```python
from build123d import *

# Parameters (mm, degrees)
SKETCH2_R            = 2
BOSS_EXTRUDE1_DEPTH  = 28
SKETCH3_R            = 3
BOSS_EXTRUDE2_DEPTH  = 1
FILLET1_R            = 1
FILLET1_OF_MIRROR1_R = 1


with BuildPart() as part:
    # Sketch2 → Boss-Extrude1 (new body)
    with BuildSketch(Plane(origin=(0, 0, 0), x_dir=(0, 0, -1), z_dir=(1, 0, 0))):
        Circle(SKETCH2_R)
    extrude(amount=BOSS_EXTRUDE1_DEPTH)

    # Sketch3 → Boss-Extrude2 (add)
    with BuildSketch(Plane(origin=(28, 0, 0), x_dir=(0, 0, -1), z_dir=(1, 0, 0))):
        Circle(SKETCH3_R)
    boss_extrude2 = extrude(amount=BOSS_EXTRUDE2_DEPTH)

    # Fillet1
    fillet1_edges = [part.edges().sort_by_distance(p)[0] for p in [
        (29, 0, 3),
    ]]
    fillet(fillet1_edges, radius=FILLET1_R - 0.0001)  # a hair under: the kernel refuses the full size

    # Mirror1: Boss-Extrude2 across plane
    add(boss_extrude2.mirror(Plane.ZY.offset(-14)))

    # Fillet1 of Mirror1
    fillet1_of_mirror1_edges = [part.edges().sort_by_distance(p)[0] for p in [
        (-1, 0, 3),
    ]]
    fillet(fillet1_of_mirror1_edges, radius=FILLET1_OF_MIRROR1_R - 0.0001)  # a hair under: the kernel refuses the full size


solid = part.part
```
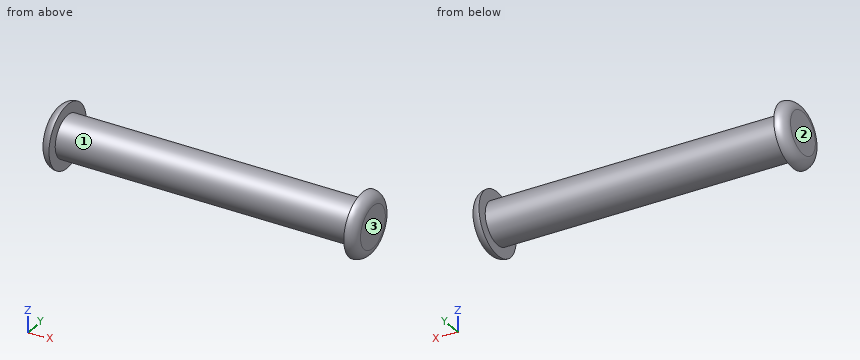
CAD build for the part. Positions are in the model's coordinates, mm. Face numbers are marked on the shaded views. Round coordinates to 2 decimals unless told otherwise and drop trailing zeros. Order: outer loops, then holes, each group sorted by start corner. A loop starts at its lowest first (then second) coordinate and runs counter-clockwise, first axis right, second up. Notation, with made-up numbers: (-34.75, 52) - (22.25, 52) arc R32 ccw to (22.25, 91) - close; hole circle Ø5 at (51, -18.75). An arc over 180 degrees is marked (long way). Answer in a Markdown table with one row per item. Add a question column.
(1) Band-saw the part on C-C on x = 18. List the corners of the cut face in (y, z), and give its area (3 significant figures).
(2) Probe L1, parallel to X at y = 0, z = -2.1 (3 decimals); L2, parallel to Y at x = 25.5, z = -0.1; L3, parallel to X at y = 1.25, z = 2.6. List the from-to ranges inside material, lowest first. Write a range as [from, to].
(3) Mould opens along X. For the marked faces 1, 2 and 3 say: +X half, -X half, draft (parallel to the pull), parting line (faces both ways), or undercut.
(4) Drop flat-ended pins along their axis: pin 1 Ø3 at (y, z) = (-1.5, -1.5) entering from -X; pin 2 Ø1 at (x, y) = (24, -0.5) entering from +Z; pin 3 Ø1.5 at (x, y) = (6, -2.5) entering from +Z; pin 4 Ø1.5 at (x, z) = (21, 1) entering from +Y. Give the stop position or say it passes through.
Data:
| question | item | result |
|---|---|---|
| 1 | outline | circle Ø4 at (0, 0) |
| 1 | area | 12.6 mm^2 |
| 2 | L1 | x = [-0.995, 0], [28, 28.995] |
| 2 | L2 | y = [-2, 2] |
| 2 | L3 | x = [-0.47, 0], [28, 28.47] |
| 3 | face 1 | undercut |
| 3 | face 2 | -X half |
| 3 | face 3 | +X half |
| 4 | pin 1 | stops at x = -1 |
| 4 | pin 2 | stops at z = 2 |
| 4 | pin 3 | stops at z = 0.97 |
| 4 | pin 4 | stops at y = 1.98 |
